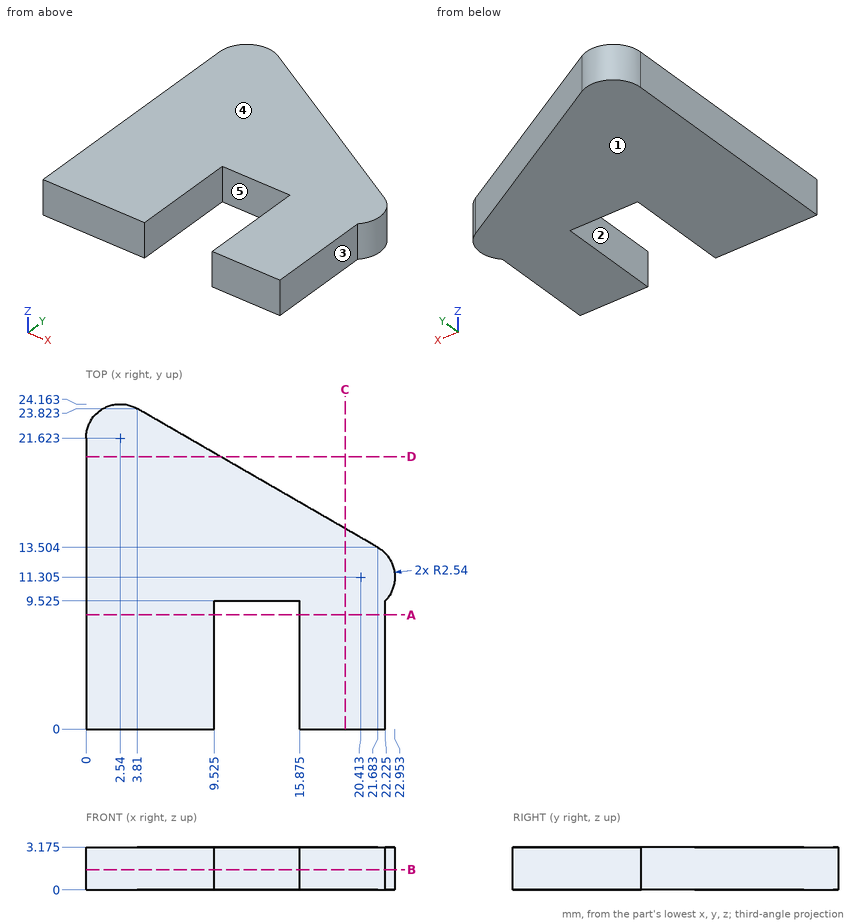
Could you check a few things on this drawing? It's one solid part, dimensions in mm from its lowest x, y, z. A direction names the side the tool comes from. Give positions to 0.01 mm unless a question says otherwise; leave off trailing zeros. Write each loop counter-clockwise with the first axis right and the second up, starting at its lowest first coordinate (ties: lowest second). Pieces come first, ordered by that corner, then holes. Notation, with made-up numbers: M -39,-39 L -1,-39 A10 cw -1,-25 Z; hole C 16,57 d6. An arc over 180 degrees is marked long. Put each result on its own line as item: value. Start each with the question number.
Item 1: If we section it at A-A, the plane y = 8.5: Write out the boundary of the cut face in (x, z) (1 decimal).
Item 2: If we section it at D-D, the plane y = 20.25: Write out the boundary of the cut face in (x, z) (1 decimal).
Item 3: Will these pins go through, and if not, where does the flat tip stop? pin 1 (1 mm diameter, centred on x = 13.5, z = 1.5, fed in from -Y) (3 decimals); pin 2 (1 mm diameter, centred on y = 21, z = 2, fed in from +X) (1 decimal); pin 3 (1 mm diameter, centred on y = 7, z = 1.5, fed in from +X) (3 decimals).
Item 4: If we section it at C-C, the plane x = 19.25: Write out the boundary of the cut face in (y, z) (1 decimal).
Item 5: Thinking about a two-plate mould opening in X: for the marked faces 1, 2 and 3, which applies, +X half, -X half, draft (parallel to the pull), parting line (faces both ways), or undercut?
Item 6: If we section it at B-B, the plane z = 1.5: Write out the boundary of the cut face in (x, y) (1 decimal), then the cut area to 3 significant figures.
Item 7: On a 3-axis mill with a long thin cutter (end or side, diameter ignored), from which of +Z, -Z, +X, -X, +Y, -Y can I reach the whole of each face in a straight line? I mean the marked faces 4 and 5. Say none if no direction works.
Item 8: I need wall thicknesses on L1, parallel to X at y = 6.5, z = 0.8 (1 decimal); L2, parallel to Y at x = 14.25, z = 2.15 (1 decimal); L3, parallel to Y at x = 6, z = 1.4. Which ranges of each line are inside material? Lowest first, please. Write a range as from..to.
Values:
1. outline: M 0,0 L 9.5,0 L 9.5,3.2 L 0,3.2 Z; M 15.9,0 L 22.2,0 L 22.2,3.2 L 15.9,3.2 Z
2. outline: M 0,0 L 10,0 L 10,3.2 L 0,3.2 Z
3. pin 1: y = 9.525
3. pin 2: x = 9.6
3. pin 3: x = 22.225
4. outline: M 0,0 L 14.9,0 L 14.9,3.2 L 0,3.2 Z
5. face 1: draft
5. face 2: undercut
5. face 3: +X half
6. outline: M 0,0 L 9.5,0 L 9.5,9.5 L 15.9,9.5 L 15.9,0 L 22.2,0 L 22.2,9.5 A2.5 ccw 21.7,13.5 L 3.8,23.8 A2.5 ccw 0,21.6 Z
6. area: 373 mm²
7. face 4: +Z, +X, -X, +Y, -Y
7. face 5: +Z, -Z, -Y
8. L1: 0..9.5, 15.9..22.2
8. L2: 9.5..17.8
8. L3: 0..22.56
